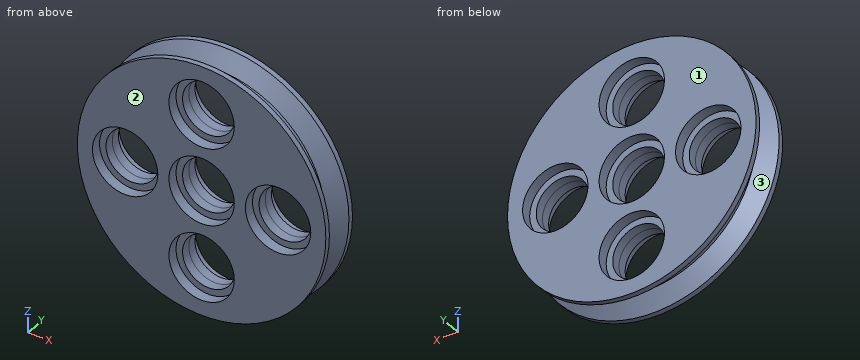
```python
from build123d import *

# Parameters (mm, degrees)
HOLE1_D           = 4
HOLE1_DEPTH       = 1.5
HOLE1_CBORE_D     = 5
HOLE1_CBORE_DEPTH = 0.8
HOLE1_TIP         = 1.201721238


with BuildPart() as part:
    # Sketch2 → Revolve1 (revolve)
    with BuildSketch(Plane.XY):
        Polygon((9.5, 0.75), (9.5, 0.35), (8.300666852, -0.5), (8.300666852, -0.75), (0, -0.75), (0, 0.75), align=None)
    revolve(axis=Axis((0, 0.75, 0), (0, -1, 0)))

    # Hole1
    with Locations(Plane(origin=(0, 0.75, 0), x_dir=(1, 0, 0), z_dir=(0, 1, 0))):
        with Locations((0, 0), (-5.85, 0), (5.85, 0), (0, 5.85), (0, -5.85)):
            CounterBoreHole(HOLE1_D / 2, HOLE1_CBORE_D / 2, HOLE1_CBORE_DEPTH, depth=HOLE1_DEPTH)
            with Locations((0, 0, -(HOLE1_DEPTH + HOLE1_TIP / 2))):  # 118° drill point
                Cone(0, HOLE1_D / 2, HOLE1_TIP, mode=Mode.SUBTRACT)

    # Mirror1: part across plane


with BuildPart() as part_1:
    add(part.part)
    add(part.part.mirror(Plane.ZX.offset(-0.75)))


solid = part_1.part
```
Geometry: final body of the model. Coordinates: model frame, mm. Face numbers are marked on the shaded views. Round coordinates to 2 decimals unless told otherwise and drop trailing zeros. Use CSV: the item, a comma, the result in double quotes. Start each with the question number.
Q1. Section A-A (z = 0). Give the number of separate pieces and of enclosed holes in the cut face, plus the area to 3 significant figures.
Q2. First-contact query: pin 1 Ø1 at (y, z) = (-1, -4) entering from -X; pin 2 Ø3 at (x, z) = (0, 0) entering from -Y; pin 3 Ø4.5 at (x, z) = (-5.85, 0) entering from +Y; pin 4 Ø1 at (x, y) = (-0.5, -0.5) entering from +Z. Flat tips, straight axial feed; report the tip coordinate or a pass-through.
Q3. Line query: L1, parallel to Z at x = 0, y = -2; L2, parallel to X at y = -2.05, z = 1.25; L3, parallel to Z at x = -1, y = 0.4. Output: solid intervals per line, ascending.
Q4. Pull-direction query (Y, two-part tool) for the marked faces 1, 2 and 3; classes: pulls with the +Y half, pulls with the -Y half, needs draft (parallel to the pull), parting line crosses it, or undercut.
Result sheet:
1,separate pieces,"4"
1,enclosed holes,"0"
1,area,"13.0 mm²"
2,pin 1,"x = -8.11"
2,pin 2,"through"
2,pin 3,"y = -0.05"
2,pin 4,"z = 8.99"
3,L1,"-9.5 to -8.35, -3.35 to -2.5, 2.5 to 3.35, 8.35 to 9.5"
3,L2,"-9.42 to -8.02, -3.68 to -2.17, 2.17 to 3.68, 8.02 to 9.42"
3,L3,"-9.45 to -8.14, -3.56 to -2.29, 2.29 to 3.56, 8.14 to 9.45"
4,face 1,"pulls with the +Y half"
4,face 2,"pulls with the -Y half"
4,face 3,"undercut"
